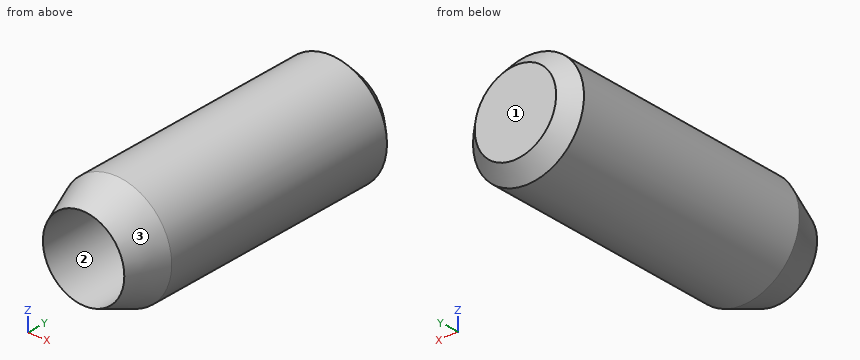
```python
from build123d import *

# Parameters (mm, degrees)
F0_R     = 19.05
F0_R_2   = 12.7
F1_DEPTH = 101.6
F2_SIZE2 = 12.7
F2_SIZE  = 5.08
F3_DEPTH = 95.25
F4_SIZE  = 5.08


with BuildPart() as f1:
    # F0 (on Front) → F1 (new body)
    with BuildSketch(Plane.XZ):
        Circle(F0_R)
        Circle(F0_R_2, mode=Mode.SUBTRACT)
        Circle(F0_R_2)
    extrude(amount=F1_DEPTH)

    # F2
    f2_edges = [f1.edges().sort_by_distance(p)[0] for p in [
        (-19.05, -101.6, 0),
    ]]
    f2_side = f1.faces().sort_by_distance((0, -101.6, 0))[0]
    chamfer(f2_edges, length=F2_SIZE, length2=F2_SIZE2, reference=f2_side)

    # F3 (cut): a face of the model
    f3_faces = [f1.faces().sort_by_distance(p)[0] for p in [
        (0, -101.6, 0),
    ]]
    extrude(f3_faces, amount=-F3_DEPTH, mode=Mode.SUBTRACT)

    # F4
    f4_edges = [f1.edges().sort_by_distance(p)[0] for p in [
        (-19.05, 0, 0),
    ]]
    chamfer(f4_edges, length=F4_SIZE)


solid = f1.part
```
Check sheet for the modelled part. Datum: model origin and axes. Units: mm. Face numbers are marked on the shaded views. Round coordinates to 2 decimals unless told otherwise and drop trailing zeros. Loops run counter-clockwise (first coordinate to the right, second up) from the corner with the lowest first, then second, coordinate; pieces in that order, holes last. Notation, with made-up numbers: (30.5, 42.25) - (60.5, 42.25) arc R15 ccw to (60.5, 51.25) - close; hole circle Ø8 at (56, -19). An arc over 180 degrees is marked (long way). Answer as a JSON object with one key per item and string values. Group by question number.
Q1. Mould release check, pull along Z, two halves, no side actions. Record for the marked faces 1, 2 and 3: released by +Z, released by -Z, zero draft, split by the parting line, or undercut.
Q2. Sectioned sample at C-C, the plane y = -20. Enter the section's corners in (x, z), plus the area to 3 significant figures.
Q3. Sectioned sample at B-B, the plane x = 0. Enter the section's corners in (y, z).
Q4. Scan lines: line 1 along Z through (x, y) = (0, -62); line 2 along X through (y, z) = (-14, -0.5); line 3 along X through (y, z) = (-20, -5.5). Record each from-to range of solid material in increasing order. Write a range as [from, to].
Q5. Sectioned sample at A-A, the plane z = 0. Enter the section's corners in (x, y), plus the area to 3 significant figures.
Q6. Gauge pin test, flat ends, axial feed: P1, Ø6, axis at x = -11, z = 3, coming from the -Y side; P2, Ø2, axis at x = -4, y = -89, coming from the -Z side; P3, Ø22.5, axis at x = -0.5, z = 1, coming from the -Y side; P4, Ø1.5, axis at y = -39, z = -6.5, coming from the +X side. Record the tip position at first contact, or that the pin passes through.
Solution:
{
 "1": {"face 1": "zero draft", "face 2": "undercut", "face 3": "split by the parting line"},
 "2": {"outline": "circle Ø38.1 at (0, 0); hole circle Ø27.94 at (0, 0)", "area": "527 mm²"},
 "3": {"outline": "(-101.6, -13.97) - (-88.9, -19.05) - (-5.08, -19.05) - (0, -13.97) - (0, 13.97) - (-5.08, 19.05) - (-88.9, 19.05) - (-101.6, 13.97) - (-6.35, 13.97) - (-6.35, -13.97) - close"},
 "4": {"line 1": "z = [-19.05, -13.97], [13.97, 19.05]", "line 2": "x = [-19.04, -13.96], [13.96, 19.04]", "line 3": "x = [-18.24, -12.84], [12.84, 18.24]"},
 "5": {"outline": "(-19.05, -88.9) - (-13.97, -101.6) - (-13.97, -6.35) - (13.97, -6.35) - (13.97, -101.6) - (19.05, -88.9) - (19.05, -5.08) - (13.97, 0) - (-13.97, 0) - (-19.05, -5.08) - close", "area": "1,120 mm²"},
 "6": {"P1": "stops at y = -101.6", "P2": "stops at z = -18.81", "P3": "stops at y = -6.35", "P4": "stops at x = 18.16"}
}
